Verification items for the finished model (mm, model axes). A direction names the side the tool comes from. Round coordinates to 2 decimals unless told otherwise and drop trailing zeros. Write each loop counter-clockwise with the first axis right and the second up, starting at its lowest first coordinate (ties: lowest second). Pieces come first, ordered by that corner, then holes. Notation, with made-up numbers: M 83.5,-10.5 L 101.5,-10.5 A19 cw 101.5,-0.5 Z; hole C -6.75,-37 d3. An arc over 180 degrees is marked long. Write each question's results on one line, items separated by ' | '.
from build123d import *

# Parameters (mm, degrees)
SKETCH2_R          = 2
CUT_EXTRUDE1_DEPTH = 10


with BuildPart() as part:
    # Sketch1 → Revolve1 (revolve)
    with BuildSketch(Plane.XY):
        Polygon((17.5, 60.5), (13, 60.5), (13, 61.5), (8, 61.5), (8, 20.5), (0, 20.5), (0, 0), (52, 0), (61.5, 11), (67.5, 11), (67.5, 15.5), (63, 15.5), (63, 51.5), (67.5, 51.5), (67.5, 56.5), (25, 56.5), align=None)
    revolve(axis=Axis((0, 20.5, 0), (0, -1, 0)))

    # Sketch2 → Cut-Extrude1 (cut)
    with BuildSketch(Plane.XZ):
        with Locations((0, 27.5)):
            Circle(SKETCH2_R)
        with Locations((19.445436483, 19.445436483)):
            Circle(SKETCH2_R)
        with Locations((27.5, 0)):
            Circle(SKETCH2_R)
        with Locations((19.445436483, -19.445436483)):
            Circle(SKETCH2_R)
        with Locations((0, -27.5)):
            Circle(SKETCH2_R)
        with Locations((-19.445436483, -19.445436483)):
            Circle(SKETCH2_R)
        with Locations((-27.5, 0)):
            Circle(SKETCH2_R)
        with Locations((-19.445436483, 19.445436483)):
            Circle(SKETCH2_R)
    extrude(amount=-CUT_EXTRUDE1_DEPTH, mode=Mode.SUBTRACT)


solid = part.part
1) Sectioned sample at A-A, the plane y = 45.5. Record the cut outline in (x, z).
Calculated:
outline: C 0,0 d126; hole C 0,0 d16
2) Draft check along X on faces 5 (the cylindrical face through (-53.57, 13.28, -41.07)), 6 (the flat face through (-3, 60.5, 13)), 7 (the flat face through (0, 10, 28)). Enter one of: pulls with the +X half, pulls with the -X half, needs draft (parallel to the pull), parting line crosses it, or undercut.
Calculated:
face 5: parting line crosses it | face 6: needs draft | face 7: undercut
3) Material ranges on line 1 (Y direction, x = -41, z = -13.5); line 2 (Y direction, x = -31.5, z = 53.5); line 3 (Z direction, x = -4.5, y = 58.5), recorded low to high. Write a range as [from, to].
Calculated:
line 1: y = [0, 56.5] | line 2: y = [11, 56.5] | line 3: z = [-20.77, -6.61], [6.61, 20.77]
4) Depth check by flat-ended pin: P1, Ø12, axis at x = 41.5, z = 45, coming from the +Y side; P2, Ø10, axis at y = 20, z = -1, coming from the -X side; P3, Ø6, axis at x = 17, y = 55, coming from the -Z side; P4, Ø5, axis at x = -22, z = 7.5, coming from the +Y side. Enter the tip coordinate at first touch or a pass-through.
Calculated:
P1: stops at y = 56.5 | P2: stops at x = -67.5 | P3: stops at z = -66.03 | P4: stops at y = 58.77
5) Access from +Z, -Z, +X, -X, +Y, -Y to the whole of each face (thin tool, end or side, straight path). Record for faces 1 (the flat face through (0, 10, -27)), 2 (the cylindrical face through (-53.57, 54.04, -41.07)), 3 (the flat face through (0, 20.5, 0)), 4 (the cylindrical face through (-8.201, 33.752, 62.464)).
Calculated:
face 1: -Y | face 2: +Y, -Y | face 3: +Y | face 4: none
